CAD build for the part. Positions are in the model's coordinates, mm. Face numbers are marked on the shaded views. A direction names the side the tool comes from. Coordinates: 2 decimals unless noted, no trailing zeros. Loops run counter-clockwise (first coordinate to the right, second up) from the corner with the lowest first, then second, coordinate; pieces in that order, holes last. Notation, with made-up numbers: (34.5, 69.5) -> (81.5, 69.5) arc R24 cw to (81.5, 108.5) -> close; hole circle Ø5 at (58, 34). An arc over 180 degrees is marked (long way). Return JSON: item names as keys, results as strings. Group by question number.
(1) Saw through at C-C on x = 2.75. Write the cut outline in (y, z).
(2) Probe L1, parallel to Y at x = -10.4, z = -3; L2, parallel to Z at x = 3.25, y = -5; L3, parallel to X at y = 0, z = 1.75. List the from-to ranges inside material, lowest first.
(3) Flat gauge pins, fed straight in: pin 1 Ø0.9 at (x, z) = (-1, 1.5) entering from -Y; pin 2 Ø2.5 at (x, z) = (11.5, -2) entering from +Y; pin 3 Ø1.4 at (x, z) = (-1.5, -7) entering from +Y. Where does each tip first touch, or does it go through?
(4) Saw through at B-B on z = -0.5. Write the cut outline in (x, y).
(5) Saw through at A-A on y = 0. Write the cut outline in (x, z).
(6) Tool access for the marked faces 1, 2 and 3: list every direction of +Z, -Z, +X, -X, +Y, -Y with a clear straight run to the whole face (end or side of a thin tool).
(7) Saw through at D-D on z = -5.75. Write the cut outline in (x, y), then the cut area to 3 significant figures.
```python
from build123d import *

# Parameters (mm, degrees)
PAD_DEPTH      = 3
PAD_DEPTH_BACK = 8.7
SKETCH001_R    = 1.05
PAD001_DEPTH   = 4


with BuildPart() as part:
    # Sketch → Pad (new body, two sides)
    with BuildSketch(Plane.XY) as pad_sk:
        with BuildLine():
            Line((-7.75, -4), (-7.75, 4))
            Line((-7.75, 4), (4.75, 4))
            ThreePointArc((7.75, 1), (6.87132, 3.12132), (4.75, 4))
            Line((7.75, 1), (7.75, -1))
            ThreePointArc((4.75, -4), (6.87132, -3.12132), (7.75, -1))
            Line((4.75, -4), (-7.75, -4))
        make_face()
    extrude(amount=PAD_DEPTH)
    extrude(pad_sk.sketch, amount=-PAD_DEPTH_BACK)

    # Sketch001 → Pad001 (join)
    with BuildSketch(Plane.XY):
        Polygon((-13.5, 4), (-13.5, -4), (-10.3, -4), (-8.5, -6), (8.5, -6), (10.3, -4), (13.5, -4), (13.5, 4), (10.3, 4), (8.5, 6), (-8.5, 6), (-10.3, 4), align=None)
        with Locations((-10.4, 0)):
            Circle(SKETCH001_R, mode=Mode.SUBTRACT)
        with Locations((10.4, 0)):
            Circle(SKETCH001_R, mode=Mode.SUBTRACT)
    extrude(amount=-PAD001_DEPTH)


solid = part.part
```
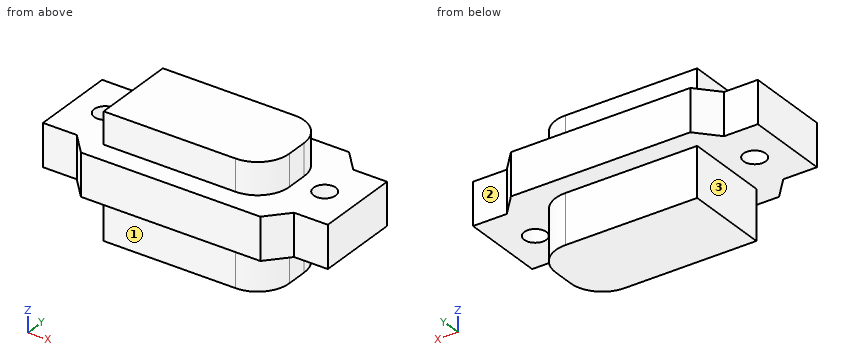
Geometry results:
{
 "1": {"outline": "(-6, -4) -> (-4, -4) -> (-4, -8.7) -> (4, -8.7) -> (4, -4) -> (6, -4) -> (6, 0) -> (4, 0) -> (4, 3) -> (-4, 3) -> (-4, 0) -> (-6, 0) -> close"},
 "2": {"L1": "-4 to -1.05, 1.05 to 4", "L2": "-4 to 0", "L3": "-7.75 to 7.75"},
 "3": {"pin 1": "y = -4", "pin 2": "y = 4.06", "pin 3": "y = 4"},
 "4": {"outline": "(-13.5, -4) -> (-10.3, -4) -> (-8.5, -6) -> (8.5, -6) -> (10.3, -4) -> (13.5, -4) -> (13.5, 4) -> (10.3, 4) -> (8.5, 6) -> (-8.5, 6) -> (-10.3, 4) -> (-13.5, 4) -> close; hole circle Ø2.1 at (-10.4, 0); hole circle Ø2.1 at (10.4, 0)"},
 "5": {"outline": "(-13.5, -4) -> (-11.45, -4) -> (-11.45, 0) -> (-13.5, 0) -> close; (-9.35, -4) -> (-7.75, -4) -> (-7.75, -8.7) -> (7.75, -8.7) -> (7.75, -4) -> (9.35, -4) -> (9.35, 0) -> (7.75, 0) -> (7.75, 3) -> (-7.75, 3) -> (-7.75, 0) -> (-9.35, 0) -> close; (11.45, -4) -> (13.5, -4) -> (13.5, 0) -> (11.45, 0) -> close"},
 "6": {"face 1": "-Z, +X, -X, -Y", "face 2": "+Z, -Z, +X, +Y", "face 3": "-Z, -X, +Y, -Y"},
 "7": {"outline": "(-7.75, -4) -> (4.75, -4) arc R3 ccw to (7.75, -1) -> (7.75, 1) arc R3 ccw to (4.75, 4) -> (-7.75, 4) -> close", "area": "120 mm²"}
}
